Part print with two shaded views. Sizes in mm from the minimum x, y, z corner. Give positions to 0.01 mm unless a question says otherwise; leave off trailing zeros. Write each loop counter-clockwise with the first axis right and the second up, starting at its lowest first coordinate (ties: lowest second). Pieces come first, ordered by that corner, then holes. Notation, with made-up numbers: (-23.5, 54) -> (29.5, 54) arc R30 ccw to (29.5, 85) -> close; hole circle Ø9 at (-4.75, 48). An arc over 180 degrees is marked (long way). Answer as a JSON object with one key per item and string values.
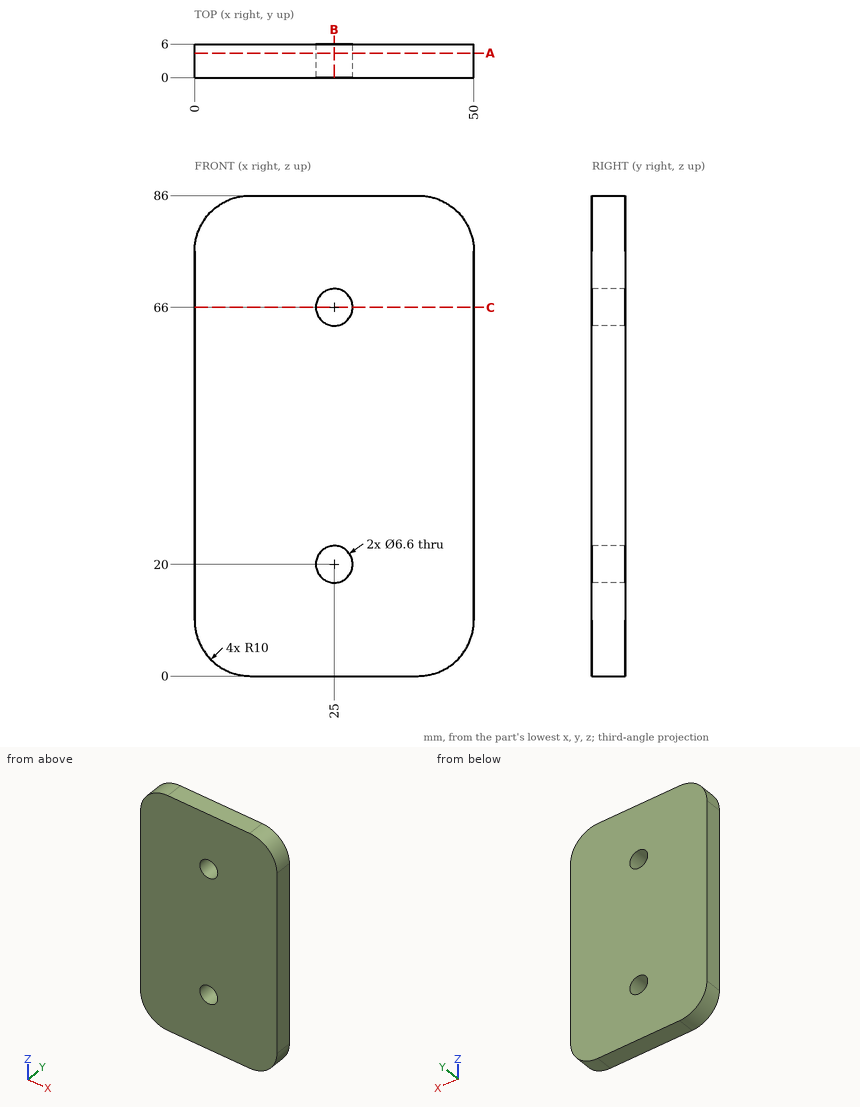
1) Slice it at C-C (z = 66). List the corners of the cut face in (x, y), then the cut area to 3 significant figures.
Model answer:
{"outline": "(0, 0) -> (21.7, 0) -> (21.7, 6) -> (0, 6) -> close; (28.3, 0) -> (50, 0) -> (50, 6) -> (28.3, 6) -> close", "area": "260 mm2"}
2) Slice it at B-B (x = 25). List the corners of the cut face in (y, z).
Model answer:
{"outline": "(0, 0) -> (6, 0) -> (6, 16.7) -> (0, 16.7) -> close; (0, 23.3) -> (6, 23.3) -> (6, 62.7) -> (0, 62.7) -> close; (0, 69.3) -> (6, 69.3) -> (6, 86) -> (0, 86) -> close"}
3) Slice it at A-A (y = 4.35). List the corners of the cut face in (x, z).
Model answer:
{"outline": "(0, 10) arc R10 ccw to (10, 0) -> (40, 0) arc R10 ccw to (50, 10) -> (50, 76) arc R10 ccw to (40, 86) -> (10, 86) arc R10 ccw to (0, 76) -> close; hole circle Ø6.6 at (25, 20); hole circle Ø6.6 at (25, 66)"}
4) Wall check: probe 1 along Z at (x, y) = (25, 1.5); probe 2 along X at (y, z) = (1.55, 22); probe 3 along X at (y, z) = (0.7, 65). Give the ranges that are in metal, low to high.
Model answer:
{"probe 1": "z = 0 to 16.7, 23.3 to 62.7, 69.3 to 86", "probe 2": "x = 0 to 22.38, 27.62 to 50", "probe 3": "x = 0 to 21.86, 28.14 to 50"}
